Verification items for the finished model (mm, model axes). Face numbers are marked on the shaded views. A direction names the side the tool comes from. Round coordinates to 2 decimals unless told otherwise and drop trailing zeros. Write each loop counter-clockwise with the first axis right and the second up, starting at its lowest first coordinate (ties: lowest second). Pieces come first, ordered by that corner, then holes. Notation, with made-up numbers: (-13, 13) - (6, 13) arc R7 cw to (6, 20) - close; hole circle Ø7 at (-13, -25). An arc over 180 degrees is marked (long way). Write each question's results on one line, items separated by ' | '.
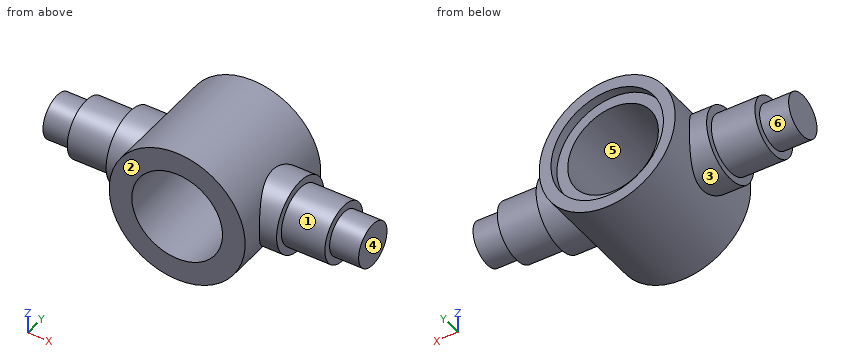
```python
from build123d import *

# Parameters (mm, degrees)
SKETCH2_R           = 37.5
BOSS_EXTRUDE1_DEPTH = 32
HOLE1_D             = 50
HOLE1_CBORE_D       = 62
HOLE1_CBORE_DEPTH   = 5


with BuildPart() as part:
    # Sketch1 → Revolve1 (revolve)
    with BuildSketch(Plane(origin=(0, 0, 0), x_dir=(1, 0, 0), z_dir=(0, 1, 0)), mode=Mode.PRIVATE) as revolve1_sk:
        Polygon((-87, 0), (-87, 12), (-71, 12), (-71, 16), (-47, 16), (-47, 20), (47, 20), (47, 16), (71, 16), (71, 12), (87, 12), (87, 0), align=None)
    revolve(revolve1_sk.sketch.rotate(Axis((-87, 0, 0), (1, 0, 0)), 180), axis=Axis((-87, 0, 0), (1, 0, 0)))

    # Sketch2 → Boss-Extrude1 (add, symmetric)
    with BuildSketch(Plane(origin=(0, 0, 0), x_dir=(1, 0, 0), z_dir=(0, 1, 0))):
        with Locations(Location((0, 0, 0), (0, 0, 270))):
            Circle(SKETCH2_R)
    extrude(amount=BOSS_EXTRUDE1_DEPTH, both=True)

    # Hole1 (through all)
    with Locations(Plane(origin=(0, 32, 0), x_dir=(1, 0, 0), z_dir=(0, 1, 0))):
        with Locations((0, 0)):
            CounterBoreHole(HOLE1_D / 2, HOLE1_CBORE_D / 2, HOLE1_CBORE_DEPTH)


solid = part.part
```
(1) Mould release check, pull along Z, two halves, no side actions. Record for the marked faces 4, 5 and 6: released by +Z, released by -Z, zero draft, split by the parting line, or undercut.
Answer:
face 4: zero draft | face 5: undercut | face 6: split by the parting line
(2) Section check C-C (y = -26). Record the cut outline in (x, z), plus the area to 3 significant figures.
Answer:
outline: circle Ø75 at (0, 0); hole circle Ø50 at (0, 0) | area: 2,450 mm2
(3) Go/stop test with flat-tipped pins: pin 1 Ø3 at (y, z) = (-13, -25) entering from +X; pin 2 Ø1.5 at (x, y) = (-2, -21.5) entering from +Z; pin 3 Ø2 at (x, y) = (49.5, 19) entering from -Z; pin 4 Ø3 at (x, z) = (-42, 1) entering from +Y. Record where each tip stops, or that it passes through.
Answer:
pin 1: x = 29.22 | pin 2: z = 37.48 | pin 3: through | pin 4: y = 20
(4) Thickness scan on L1, parallel to Y at x = 55.5, z = 0.5; L2, parallel to Y at x = -20.5, z = -20; L3, parallel to X at y = -28, z = -23. Record the ranges inside material, lowest first.
Answer:
L1: -15.99 to 15.99 | L2: -32 to 27 | L3: -29.62 to -9.8, 9.8 to 29.62
(5) Section check D-D (x = 49.5). Record the cut outline in (y, z), plus the area to 3 significant figures.
Answer:
outline: circle Ø32 at (0, 0) | area: 804 mm2
(6) Set-up check for the marked faces 1, 2 and 3: record each of +Z, -Z, +X, -X, +Y, -Y from which the full face is reachable in a straight line by a thin tool's end or side.
Answer:
face 1: +X | face 2: +Z, -Z, +X, -X, -Y | face 3: -X
(7) Section check B-B (z = -22). Record the cut outline in (x, y), plus the area to 3 significant figures.
Answer:
outline: (-30.37, -32) - (-11.87, -32) - (-11.87, 27) - (-21.84, 27) - (-21.84, 32) - (-30.37, 32) - close; (11.87, -32) - (30.37, -32) - (30.37, 32) - (21.84, 32) - (21.84, 27) - (11.87, 27) - close | area: 2,270 mm2
(8) Section check A-A (x = 2). Record the cut outline in (y, z).
Answer:
outline: (-32, -37.45) - (32, -37.45) - (32, -30.94) - (27, -30.94) - (27, -24.92) - (-32, -24.92) - close; (-32, 24.92) - (27, 24.92) - (27, 30.94) - (32, 30.94) - (32, 37.45) - (-32, 37.45) - close
